Geometry: final body of the model. Coordinates: model frame, mm. A direction names the side the tool comes from. Coordinates: 2 decimals unless noted, no trailing zeros. Write item = value, one per line. Start each with the question number.
```python
from build123d import *

# Parameters (mm, degrees)
BOX001_W     = 30.5
BOX001_H     = 30
BOX001_DEPTH = 22
BOX002_W     = 36.5
BOX002_H     = 28
BOX002_DEPTH = 22


with BuildPart() as cube001:
    # Box001 → Box001 (new body)
    with BuildSketch(Plane.XY):
        with Locations((15.25, 15)):
            Rectangle(BOX001_W, BOX001_H)
    extrude(amount=BOX001_DEPTH)


with BuildPart() as switch_slot:
    # Box002 → Box002 (new body)
    with BuildSketch(Plane(origin=(-3, 2, 0), x_dir=(1, 0, 0), z_dir=(0, 0, 1))):
        with Locations((18.25, 14)):
            Rectangle(BOX002_W, BOX002_H)
    extrude(amount=BOX002_DEPTH)

    # Fusion001: union Cube001
    add(cube001.part)


with BuildPart() as switch_slot_1:
    # Fusion001 placement: moved
    add(switch_slot.part.moved(Location((4.75, 0, 2))))


solid = switch_slot_1.part
```
Item 1: First-contact query: pin 1 (0.9 mm diameter, centred on x = 37.5, z = 17, fed in from -Y); pin 2 (1 mm diameter, centred on y = 1, z = 17, fed in from -X). Flat tips, straight axial feed; report the tip coordinate or a pass-through.
Item 2: Material intervals for probe 1 along Y at (x, z) = (36.5, 6.75), sorted ascending. Write a range as [from, to].
Item 3: Reachability of faces 1 (the flat face through (37, 2, 13)), 2 (the flat face through (4.75, 1, 13)), 3 (the flat face through (38.25, 16, 13)) from +Z, -Z, +X, -X, +Y, -Y: full face, straight path, thin tool, end or side. Return the list, or none.
Ans:
q1.pin_1 = 2
q1.pin_2 = 4.75
q2.probe_1 = [2, 30]
q3.face_1 = +Z, -Z, +X, -Y
q3.face_2 = +Z, -Z, -X, -Y
q3.face_3 = +Z, -Z, +X, +Y, -Y
